For this review, use the dimensioned drawing (mm, ordinates from the lowest corner) and the shaded views. A direction names the side the tool comes from. Coordinates: 2 decimals unless noted, no trailing zeros. Loops run counter-clockwise (first coordinate to the right, second up) from the corner with the lowest first, then second, coordinate; pieces in that order, holes last. Notation, with made-up numbers: (-26.75, 14.25) - (28.25, 14.25) arc R22 ccw to (28.25, 37.25) - close; hole circle Ø10 at (31.25, -8). An arc over 180 degrees is marked (long way). Use one line per item in the form item = value. Start each with the question number.
(1) Add section C-C (y = 8.15). State the section outline as (x, z) points.
(2) Add section D-D (x = 17.75). State the section outline as (y, z) points.
(3) The part is to be moulded in two halves that separate along Y. For the marked faces 1, 2 and 3, say which applies: pulls with the +Y half, pulls with the -Y half, needs draft (parallel to the pull), parting line crosses it, or undercut.
(4) Add section B-B (x = 2.5). State the section outline as (y, z) points.
(5) For L1, parallel to Y at x = 2.65, z = 10; L2, parallel to Y at x = 6.25, z = 13.75; L3, parallel to X at y = 3, z = 10.25, list the stretches that pass through material, from the lowest coordinate up.
(6) Tool access review of the marked faces 4, 5 and 6: name each direction out of +Z, -Z, +X, -X, +Y, -Y from which nothing blocks a thin tool from reaching the whole face with its end or side.
(7) Clearance check with flat-ended pins moving along their axes: pin 1 Ø1.5 at (x, y) = (13.5, 5) entering from +Z; pin 2 Ø6 at (y, z) = (11, 9.5) entering from -X. State where each tip first meets the part, or that it passes through.
(8) Add section A-A (z = 10). State the section outline as (x, y) points, plus the area to 3 significant figures.
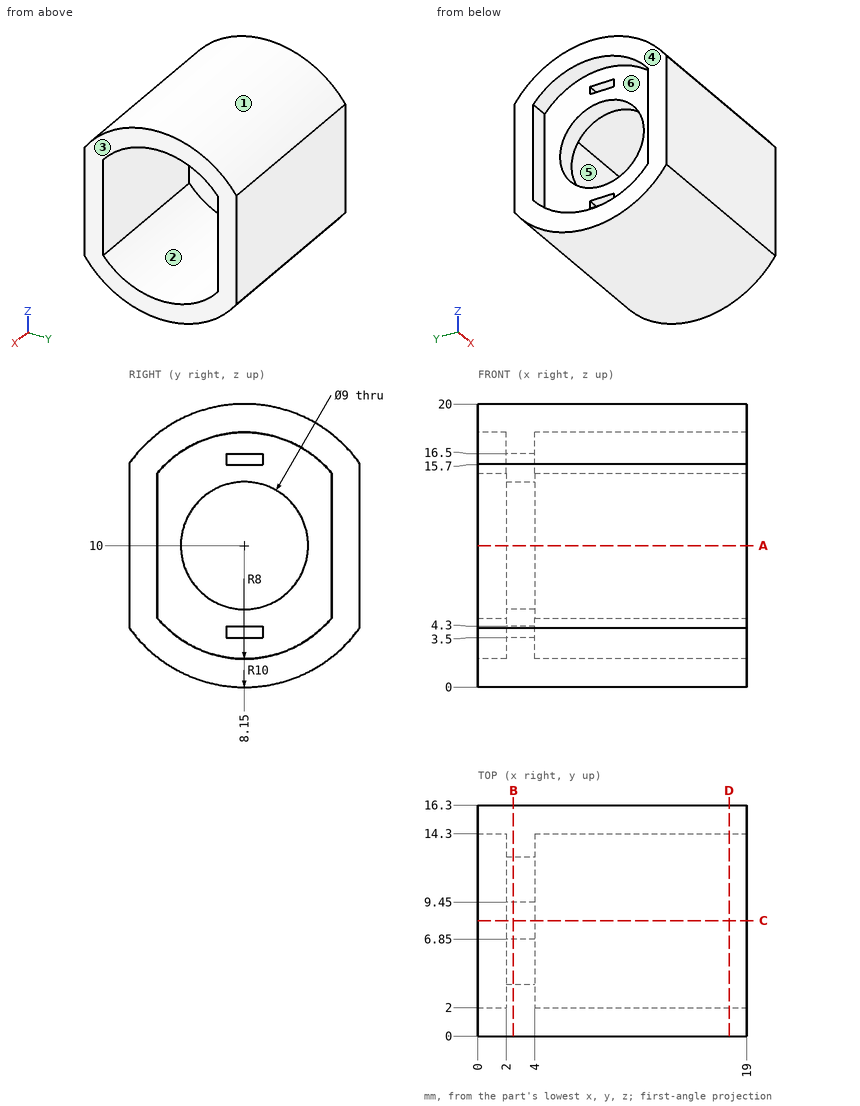
Computed values:
q1.outline = (0, 0) - (19, 0) - (19, 2) - (4, 2) - (4, 3.5) - (2, 3.5) - (2, 2) - (0, 2) - close; (0, 18) - (2, 18) - (2, 16.5) - (4, 16.5) - (4, 18) - (19, 18) - (19, 20) - (0, 20) - close; (2, 4.3) - (4, 4.3) - (4, 5.5) - (2, 5.5) - close; (2, 14.5) - (4, 14.5) - (4, 15.7) - (2, 15.7) - close
q2.outline = (0, 4.21) arc R10 ccw to (16.3, 4.21) - (16.3, 15.79) arc R10 ccw to (0, 15.79) - close; hole (2, 4.88) arc R8 ccw to (14.3, 4.88) - (14.3, 15.12) arc R8 ccw to (2, 15.12) - close
q3.face_1 = parting line crosses it
q3.face_2 = undercut
q3.face_3 = needs draft
q4.outline = (0, 4.21) arc R10 ccw to (16.3, 4.21) - (16.3, 15.79) arc R10 ccw to (0, 15.79) - close; hole circle Ø9 at (8.15, 10); hole (6.85, 3.5) - (9.45, 3.5) - (9.45, 4.3) - (6.85, 4.3) - close; hole (6.85, 15.7) - (9.45, 15.7) - (9.45, 16.5) - (6.85, 16.5) - close
q5.L1 = 0 to 3.65, 12.65 to 16.3
q5.L2 = 0 to 2, 14.3 to 16.3
q5.L3 = 2 to 4
q6.face_4 = +Z, -Z, -X, +Y, -Y
q6.face_5 = +X
q6.face_6 = -X
q7.pin_1 = 19.71
q7.pin_2 = 2
q8.outline = (0, 0) - (19, 0) - (19, 2) - (4, 2) - (4, 3.65) - (2, 3.65) - (2, 2) - (0, 2) - close; (0, 14.3) - (2, 14.3) - (2, 12.65) - (4, 12.65) - (4, 14.3) - (19, 14.3) - (19, 16.3) - (0, 16.3) - close
q8.area = 82.6 mm^2
